CAD build for the part. Positions are in the model's coordinates, mm. A direction names the side the tool comes from. Give positions to 0.01 mm unless a question says otherwise; leave off trailing zeros. Order: outer loops, then holes, each group sorted by start corner. A loop starts at its lowest first (then second) coordinate and runs counter-clockwise, first axis right, second up.
Item 1: Band-saw the part on B-B on z = 36. Give the cut face in (x, y), plus the area to 3 significant figures.
Item 2: Band-saw the part on C-C on z = 5.5. Count the separate pieces of the cut face and the enclosed holes in it, plus the area to 3 significant figures.
Item 3: Wall check: L1, parallel to X at y = 30, z = 5.5; L2, parallel to Z at x = -25.5, y = 19; L3, parallel to Y at x = -12.5, z = 6. Give the ranges that are in metal, low to high.
Item 4: Band-saw the part on D-D on y = 26. Give the cut face in (x, z), plus the area to 3 significant figures.
Item 5: Two-plate mould, pull along X, no slides. Class faces 3 (the cylindrical face through (0.433, 5.086, 3.644)), 4 (the flat face through (5.615, 10, 4)), 5 (the cylindrical face through (2.951, 4.405, 7.214)), 6 (the flat face through (-30.346, 10, 19)): released by +X, released by -X, zero draft, split by the parting line, or undercut.
Item 6: Which spindle directions (+Z, -Z, +X, -X, +Y, -Y) get a long thin tool onto all of the face, cutting with end or side? Do faces 1 (the cylindrical face through (-2.272, 27.535, 3.644)), 2 (the flat face through (-9, -2, 7.392)). Say none if no direction does.
Item 7: Band-saw the part on A-A on x = -6. Give the cut face in (y, z) (3 decimals).
Item 8: Flat gauge pins, fed straight in: P1, Ø3, axis at y = 14.5, z = 23.5, coming from the +X side; P2, Ø5.5, axis at x = -14.47, y = -8.31, coming from the +Z side; P3, Ø4, axis at y = 4.39, z = 22.22, coming from the -X side. Where does each tip first touch, or does it go through?
```python
from build123d import *

# Parameters (mm, degrees)
F0_W     = 7.391951
F0_H     = 44.45
F1_DEPTH = 38.1
F0_W_2   = 28.569102
F0_R     = 2.3114
F2_DEPTH = 7.391959
F3_R     = 2.3114
F4_DEPTH = 50.8


with BuildPart() as f1:
    # F0 (on Top) → F1 (new body)
    with BuildSketch(Plane.XY):
        with Locations((-26.65034, 10.741919)):
            Rectangle(F0_W, F0_H)
    extrude(amount=F1_DEPTH)

    # F0 (on Top) → F2 (join)
    with BuildSketch(Plane.XY):
        with Locations((-8.669814, 10.741919)):
            Rectangle(F0_W_2, F0_H)
        with Locations((-14.471316, -8.308081)):
            Circle(F0_R, mode=Mode.SUBTRACT)
        with Locations((-14.471316, 4.391919)):
            Circle(F0_R, mode=Mode.SUBTRACT)
        with Locations((-1.771316, -8.308081)):
            Circle(F0_R, mode=Mode.SUBTRACT)
        with Locations((-1.771316, 4.391919)):
            Circle(F0_R, mode=Mode.SUBTRACT)
        with Locations((-14.471316, 17.091919)):
            Circle(F0_R, mode=Mode.SUBTRACT)
        with Locations((-14.471316, 29.791919)):
            Circle(F0_R, mode=Mode.SUBTRACT)
        with Locations((-1.771316, 17.091919)):
            Circle(F0_R, mode=Mode.SUBTRACT)
        with Locations((-1.771316, 29.791919)):
            Circle(F0_R, mode=Mode.SUBTRACT)
    extrude(amount=F2_DEPTH)

    # F3 (on face) → F4 (cut)
    with BuildSketch(Plane(origin=(-30.346316, 0, 0), x_dir=(0, -1, 0), z_dir=(-1, 0, 0))):
        with Locations((8.308081, 34.925)):
            Circle(F3_R)
        with Locations((-4.391919, 34.925)):
            Circle(F3_R)
        with Locations((-17.091919, 34.925)):
            Circle(F3_R)
        with Locations((-29.791919, 34.925)):
            Circle(F3_R)
        with Locations((-29.791919, 22.225)):
            Circle(F3_R)
        with Locations((-17.091919, 22.225)):
            Circle(F3_R)
        with Locations((-4.391919, 22.225)):
            Circle(F3_R)
        with Locations((8.308081, 22.225)):
            Circle(F3_R)
        with Locations((8.308081, 9.525)):
            Circle(F3_R)
        with Locations((-4.391919, 9.525)):
            Circle(F3_R)
        with Locations((-17.091919, 9.525)):
            Circle(F3_R)
        with Locations((-29.791919, 9.525)):
            Circle(F3_R)
    extrude(amount=-F4_DEPTH, mode=Mode.SUBTRACT)


solid = f1.part
```
The answers:
1. outline: (-30.35, -11.48) - (-22.95, -11.48) - (-22.95, -10.35) - (-30.35, -10.35) - close; (-30.35, -6.26) - (-22.95, -6.26) - (-22.95, 2.35) - (-30.35, 2.35) - close; (-30.35, 6.44) - (-22.95, 6.44) - (-22.95, 15.05) - (-30.35, 15.05) - close; (-30.35, 19.14) - (-22.95, 19.14) - (-22.95, 27.75) - (-30.35, 27.75) - close; (-30.35, 31.84) - (-22.95, 31.84) - (-22.95, 32.97) - (-30.35, 32.97) - close
1. area: 208 mm2
2. separate pieces: 1
2. enclosed holes: 8
2. area: 1,460 mm2
3. L1: x = -30.35 to -16.77, -12.17 to -4.07, 0.53 to 5.61
3. L2: z = 0 to 8.22, 10.83 to 20.92, 23.53 to 33.62, 36.23 to 38.1
3. L3: y = -11.48 to -9.51, -7.1 to 3.19, 5.6 to 15.89, 18.3 to 28.59, 31 to 32.97
4. outline: (-30.35, 0) - (5.61, 0) - (5.61, 7.39) - (-22.95, 7.39) - (-22.95, 38.1) - (-30.35, 38.1) - close
4. area: 493 mm2
5. face 3: undercut
5. face 4: released by +X
5. face 5: zero draft
5. face 6: released by -X
6. face 1: +Z, -Z
6. face 2: +Z, +X, +Y, -Y
7. outline: (-11.483, 0) - (32.967, 0) - (32.967, 7.392) - (30.682, 7.392) arc R2.311 cw to (28.902, 7.392) - (17.982, 7.392) arc R2.311 cw to (16.202, 7.392) - (5.282, 7.392) arc R2.311 cw to (3.502, 7.392) - (-7.418, 7.392) arc R2.311 cw to (-9.198, 7.392) - (-11.483, 7.392) - close
8. P1: stops at x = -22.95
8. P2: stops at z = 7.39
8. P3: passes through
